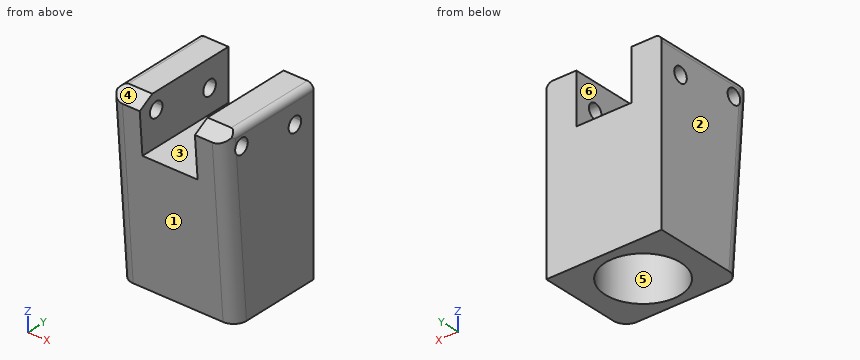
from build123d import *

# Parameters (mm, degrees)
F1_DEPTH     = 46
F3_DEPTH     = 40
F5_DEPTH     = 254
F6_W         = 22
F6_H         = 20
F7_DEPTH     = 1346.2
F8_DEPTH     = 65
F10_DEPTH    = 127
F12_DEPTH    = 254
F14_DEPTH    = 254
F15_T1_DEPTH = 103.8636030304
F15_T3_DEPTH = 103.8636030304
F17_T1_DEPTH = 49.0578822911


# Not quite as in the source:
# - a fillet or chamfer that OpenCascade refuses, or shapes differently, is made with other operations: its cross-section is extruded or revolved along the edge and cut away or added
# - a feature of the source that left no trace in its solid (it failed there, or was rolled back) is left out


with BuildPart() as f1:
    # F0 (on Right) → F1 (new body)
    with BuildSketch(Plane.YZ):
        Polygon((52, 0), (0, 0), (12, -60), (12, -70), (52, -70), align=None)
    extrude(amount=F1_DEPTH)

    # F2 (on face) → F3 (cut)
    with BuildSketch(Plane(origin=(0, 0, -70), x_dir=(1, 0, 0), z_dir=(0, 0, -1))):
        with BuildLine():
            Line((23, -33.3181476), (38, -33.3181476))
            ThreePointArc((38, -33.3181476), (12.3933982822, -22.7115458822), (23, -48.3181476))
            Line((23, -48.3181476), (23, -33.3181476))
        make_face()
        with BuildLine():
            ThreePointArc((23, -48.3181476), (33.6066017178, -43.9247493178), (38, -33.3181476))
            Line((38, -33.3181476), (23, -33.3181476))
            Line((23, -33.3181476), (23, -48.3181476))
        make_face()
    extrude(amount=-F3_DEPTH, mode=Mode.SUBTRACT)

    # F4 (on face) → F5 (cut)
    with BuildSketch(Plane.YZ.offset(46)):
        with BuildLine():
            Line((17.5, -6.5), (20.5, -6.5))
            ThreePointArc((20.5, -6.5), (19.6213203436, -4.3786796564), (17.5, -3.5))
            Line((17.5, -3.5), (17.5, -6.5))
        make_face()
        with BuildLine():
            ThreePointArc((17.5, -3.5), (15.3786796564, -8.6213203436), (20.5, -6.5))
            Line((20.5, -6.5), (17.5, -6.5))
            Line((17.5, -6.5), (17.5, -3.5))
        make_face()
    extrude(amount=-F5_DEPTH, mode=Mode.SUBTRACT)

    # F6 (on face) → F7 (cut)
    with BuildSketch(Plane(origin=(0, 52, 0), x_dir=(-1, 0, 0), z_dir=(0, 1, 0))):
        with Locations((-23, -10)):
            Rectangle(F6_W, F6_H)
    extrude(amount=-F7_DEPTH, mode=Mode.SUBTRACT)

    # F4 (on face) → F8 (cut)
    with BuildSketch(Plane.YZ.offset(46)):
        with BuildLine():
            ThreePointArc((43, -7.5), (40.8786796564, -12.6213203436), (46, -10.5))
            ThreePointArc((46, -10.5), (45.1213203436, -8.3786796564), (43, -7.5))
        make_face()
    extrude(amount=-F8_DEPTH, mode=Mode.SUBTRACT)

    # F9 (on face) → F10 (cut)
    with BuildSketch(Plane.YZ.offset(46)):
        Polygon((1.1435132474, -8.0939428881), (1.6304426827, -8.0939428881), (15.6421177089, 0), (0, 0), align=None)
    extrude(amount=-F10_DEPTH, mode=Mode.SUBTRACT)

    # F11 (on Right) → F12 (cut)
    with BuildSketch(Plane.YZ):
        Polygon((0, -70.3560113907), (14.7977182642, -70.0814500451), (9.3696815893, 0), (0, 0), align=None)
    extrude(amount=F12_DEPTH, mode=Mode.SUBTRACT)

    # F13 (on face) → F14 (cut)
    with BuildSketch(Plane.XY):
        with BuildLine():
            add(Edge.make_bspline(
                [(0, 12.6551715657), (0, 9.9420361221), (2.5992305018, 9.7406599671), (3.9225574583, 9.6255876124)],
                knots=[0, 0, 0, 0, 4.9562925603, 4.9562925603, 4.9562925603, 4.9562925603], degree=3))
            Line((0, 12.6551715657), (0, 9.539283812))
            Line((0, 9.539283812), (3.9225574583, 9.6255876124))
        make_face()
        with BuildLine():
            Line((46, 9.539283812), (46, 12.6551715657))
            add(Edge.make_bspline(
                [(46, 12.6551715657), (46, 9.9420361221), (43.4007694982, 9.7406599671), (42.0774425417, 9.6255876124)],
                knots=[0, 0, 0, 0, 4.9562925603, 4.9562925603, 4.9562925603, 4.9562925603], degree=3))
            Line((42.0774425417, 9.6255876124), (46, 9.539283812))
        make_face()
    extrude(amount=-F14_DEPTH, mode=Mode.SUBTRACT)

    # F15: fillet of radius 5.08 on 2 edges, made by hand

    # F15_s2 → F15_t1 (cut)
    with BuildSketch(Plane(origin=(0, 6.4583208178, -83.3834616235), x_dir=(1, 0, 0), z_dir=(0, -0.0772219774, 0.9970139248))):
        with BuildLine():
            ThreePointArc((0, 14.4217030153), (1.4878975516, 10.8296005669), (5.08, 9.3417030153))
            Line((5.08, 9.3417030153), (0, 9.3417030153))
            Line((0, 9.3417030153), (0, 14.4217030153))
        make_face()
    extrude(amount=F15_T1_DEPTH, mode=Mode.SUBTRACT)

    # F15_s4 → F15_t3 (cut)
    with BuildSketch(Plane(origin=(0, -1.5622319844, 20.169996876), x_dir=(1, 0, 0), z_dir=(0, 0.0772219774, -0.9970139248))):
        with BuildLine():
            ThreePointArc((40.92, -9.3417030153), (44.5121024484, -10.8296005669), (46, -14.4217030153))
            Line((46, -14.4217030153), (46, -9.3417030153))
            Line((46, -9.3417030153), (40.92, -9.3417030153))
        make_face()
    extrude(amount=F15_T3_DEPTH, mode=Mode.SUBTRACT)

    # F17: fillet of radius 2.54 on 2 edges, made by hand

    # F17_s2 → F17_t1 (cut)
    with BuildSketch(Plane.XZ.offset(-58.35)):
        with BuildLine():
            ThreePointArc((2.54, 0), (0.7439487758, -0.7439487758), (0, -2.54))
            Line((0, -2.54), (0, 0))
            Line((0, 0), (2.54, 0))
        make_face()
        with BuildLine():
            ThreePointArc((43.46, 0), (45.2560512242, -0.7439487758), (46, -2.54))
            Line((46, -2.54), (46, 0))
            Line((46, 0), (43.46, 0))
        make_face()
    extrude(amount=F17_T1_DEPTH, mode=Mode.SUBTRACT)


solid = f1.part
Geometry check sheet. Reference: the model listing, model coordinates, mm. Face numbers are marked on the shaded views. A direction names the side the tool comes from. Coordinates: 2 decimals unless noted, no trailing zeros. Order: outer loops, then holes, each group sorted by start corner. A loop starts at its lowest first (then second) coordinate and runs counter-clockwise, first axis right, second up. Notation, with made-up numbers: M -11.75,-22 L 45.25,-22 A28 ccw 45.25,-4 Z; hole C -15,33.5 d5. An arc over 180 degrees is marked long. Use CSV: the item, a comma, the result in double quotes.
Item 1: Cross-section at D-D on y = 35.5. Record the cut outline in (x, z), then the cut area to 3 significant figures.
Returned:
outline,"M 0,-70 L 8.16,-70 L 8.16,-30 L 37.84,-30 L 37.84,-70 L 46,-70 L 46,-2.54 A2.54 ccw 43.46,0 L 34,0 L 34,-20 L 12,-20 L 12,0 L 2.54,0 A2.54 ccw 0,-2.54 Z"
area,"1,590 mm2"
Item 2: Mould release check, pull along X, two halves, no side actions. Record for the marked faces 1, 2 and 3: pulls with the +X half, pulls with the -X half, needs draft (parallel to the pull), parting line crosses it, or undercut.
Returned:
face 1,"needs draft"
face 2,"pulls with the -X half"
face 3,"undercut"
Item 3: Tool access check on the marked faces 4, 5 and 6. Record the directions out of +Z, -Z, +X, -X, +Y, -Y that give a thin tool (end or side, any length) a straight path to the whole face; none if there is none.
Returned:
face 4,"+Z, +X, -X, -Y"
face 5,"-Z"
face 6,"+Z, +Y, -Y"
Item 4: Gauge pin test, flat ends, axial feed: pin 1 Ø8 at (x, z) = (17.5, -38) entering from -Y; pin 2 Ø5 at (y, z) = (16, -58) entering from -X; pin 3 Ø10 at (x, z) = (36, -34) entering from -Y; pin 4 Ø5.5 at (y, z) = (17.5, -6.5) entering from +X. Record the tip position at first contact, or that the pin passes through.
Returned:
pin 1,"stops at y = 12"
pin 2,"stops at x = 0.02"
pin 3,"stops at y = 11.62"
pin 4,"passes through"
Item 5: Cross-section at B-B on y = 26. Record the cut outline in (x, z), then the cut area to 3 significant figures.
Returned:
outline,"M 0,-70 L 9.91,-70 L 9.91,-30 L 36.09,-30 L 36.09,-70 L 46,-70 L 46,-2.54 A2.54 ccw 43.46,0 L 34,0 L 34,-20 L 12,-20 L 12,0 L 2.54,0 A2.54 ccw 0,-2.54 Z"
area,"1,730 mm2"
Item 6: Thickness scan on line 1 along X through (y, z) = (43.5, -41.5); line 2 along X through (y, z) = (40.5, -55.5); line 3 along Z through (x, y) = (42, 17). Record the ranges inside material, lowest first.
Returned:
line 1,"x = 0 to 11.99, 34.01 to 46"
line 2,"x = 0 to 9.83, 36.17 to 46"
line 3,"z = -70 to -9.46, -3.54 to 0"
Item 7: Cross-section at C-C on x = 32.5. Record the cut outline in (y, z).
Returned:
outline,"M 10.92,-20 L 14.79,-70 L 21.71,-70 L 21.71,-30 L 44.93,-30 L 44.93,-70 L 52,-70 L 52,-20 Z"
Item 8: Cross-section at A-A on x = 23. Record the cut outline in (y, z), then the cut area to 3 significant figures.
Returned:
outline,"M 10.92,-20 L 14.79,-70 L 18.32,-70 L 18.32,-30 L 48.32,-30 L 48.32,-70 L 52,-70 L 52,-20 Z"
area,"757 mm2"
